Input: part model. Units: mm. Frame: model coordinates. Coordinates: 2 decimals unless noted, no trailing zeros. Write each loop counter-clockwise with the first axis right and the second up, starting at its lowest first coordinate (ties: lowest second). Pieces come first, ordered by that corner, then holes. Notation, with made-up numbers: (47, -19) - (89, -19) arc R25 cw to (89, 11) - close; hole circle Ø6 at (13, 36.25). An arc over 180 degrees is marked (long way). One line per question, with ' | ' between items. Start each with the question number.
1) Section query A-A on x = 27. Return loops of the section in (y, z).
2) Line query: line 1 (X direction, y = -0.25, z = 11); line 2 (X direction, y = -0.25, z = 5); line 3 (X direction, y = -0.1, z = 8). Output: solid intervals per line, ascending.
3) Section query C-C on y = -0.4. Return loops of the section in (x, z).
4) Section query D-D on x = 39. Return loops of the section in (y, z).
5) First-contact query: P1, Ø5, axis at x = 17.5, z = 10, coming from the +Y side. Flat tip, straight axial feed; report the tip coordinate or a pass-through.
6) Section query B-B on z = 11.5. Return loops of the section in (x, y), and give its area (3 significant figures).
```python
from build123d import *

# Parameters (mm, degrees)
F1_DEPTH = 0.5
F4_DEPTH = 53.001


with BuildPart() as f1:
    # F0 (on Front) → F1 (new body)
    with BuildSketch(Plane.XZ):
        with BuildLine():
            Line((10.7, 18.8), (0, 0))
            Line((0, 0), (53, 0))
            Line((53, 0), (42.3, 18.8))
            Line((42.3, 18.8), (34.84, 18.8))
            Line((34.84, 18.8), (34.84, 17.3))
            ThreePointArc((34.84, 17.3), (34.312792, 16.027208), (33.04, 15.5))
            ThreePointArc((33.04, 15.5), (31.767208, 16.027208), (31.24, 17.3))
            Line((31.24, 17.3), (31.24, 18.8))
            Line((31.24, 18.8), (28.3, 18.8))
            Line((28.3, 18.8), (28.3, 17.3))
            ThreePointArc((28.3, 17.3), (27.772792, 16.027208), (26.5, 15.5))
            ThreePointArc((26.5, 15.5), (25.227208, 16.027208), (24.7, 17.3))
            Line((24.7, 17.3), (24.7, 18.8))
            Line((24.7, 18.8), (21.76, 18.8))
            Line((21.76, 18.8), (21.76, 17.3))
            ThreePointArc((21.76, 17.3), (21.232792, 16.027208), (19.96, 15.5))
            ThreePointArc((19.96, 15.5), (18.687208, 16.027208), (18.16, 17.3))
            Line((18.16, 17.3), (18.16, 18.8))
            Line((18.16, 18.8), (10.7, 18.8))
        make_face()
        with BuildLine():
            ThreePointArc((21.53, 10.88), (21.899045, 11.770955), (22.79, 12.14))
            Line((22.79, 12.14), (30.21, 12.14))
            ThreePointArc((30.21, 12.14), (31.100955, 11.770955), (31.47, 10.88))
            ThreePointArc((31.47, 10.88), (31.100955, 9.989045), (30.21, 9.62))
            Line((30.21, 9.62), (22.79, 9.62))
            ThreePointArc((22.79, 9.62), (21.899045, 9.989045), (21.53, 10.88))
        make_face(mode=Mode.SUBTRACT)
    extrude(amount=F1_DEPTH)

    # F3 (on Right) → F4 (cut, through all)
    with BuildSketch(Plane.YZ):
        Polygon((0, 2), (-0.25, 0), (0, 0), align=None)
        Polygon((-0.5, 2), (-0.5, 0), (-0.25, 0), align=None)
    extrude(amount=F4_DEPTH, mode=Mode.SUBTRACT)


solid = f1.part
```
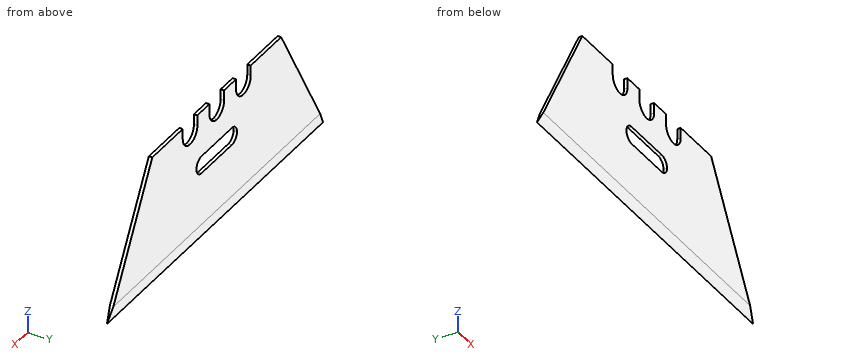
Answer key:
1) outline: (-0.5, 2) - (-0.25, 0) - (0, 2) - (0, 9.62) - (-0.5, 9.62) - close; (-0.5, 12.14) - (0, 12.14) - (0, 15.57) - (-0.5, 15.57) - close
2) line 1: 6.26 to 21.54, 31.46 to 46.74 | line 2: 2.85 to 50.15 | line 3: 4.55 to 48.45
3) outline: (0.68, 1.2) - (52.32, 1.2) - (42.3, 18.8) - (34.84, 18.8) - (34.84, 17.3) arc R1.8 cw to (33.04, 15.5) arc R1.8 cw to (31.24, 17.3) - (31.24, 18.8) - (28.3, 18.8) - (28.3, 17.3) arc R1.8 cw to (26.5, 15.5) arc R1.8 cw to (24.7, 17.3) - (24.7, 18.8) - (21.76, 18.8) - (21.76, 17.3) arc R1.8 cw to (19.96, 15.5) arc R1.8 cw to (18.16, 17.3) - (18.16, 18.8) - (10.7, 18.8) - close; hole (21.53, 10.88) arc R1.26 ccw to (22.79, 9.62) - (30.21, 9.62) arc R1.26 ccw to (31.47, 10.88) arc R1.26 ccw to (30.21, 12.14) - (22.79, 12.14) arc R1.26 ccw to start
4) outline: (-0.5, 2) - (-0.25, 0) - (0, 2) - (0, 18.8) - (-0.5, 18.8) - close
5) P1: y = 0
6) outline: (6.55, -0.5) - (21.69, -0.5) - (21.69, 0) - (6.55, 0) - close; (31.31, -0.5) - (46.45, -0.5) - (46.45, 0) - (31.31, 0) - close | area: 15.1 mm²
